Work out the finished part from the listing and answer in its coordinate system (mm). A direction names the side the tool comes from. Coordinates: 2 decimals unless noted, no trailing zeros. Order: outer loops, then holes, each group sorted by start corner. A loop starts at its lowest first (then second) coordinate and runs counter-clockwise, first axis right, second up.
1. Determine the mould class of faces 1 (the cylindrical face through (179.32, 56.47, -0.99)), 2 (the flat face through (92.93, 268, -9)), 3 (the flat face through (-142.93, 268, -9)), 4 (the flat face through (118, 292.93, -9)) for opening direction X: +X half, -X half, draft (parallel to the pull), parting line (faces both ways), or undercut.
2. Find the intervals of material crossed by probe 1 along Y at (x, z) = (0, -10.5); probe 2 along Y at (x, z) = (0, -0.7); probe 3 along Y at (x, z) = (-57, -12.5), in increasing order.
3. A tool of negligible diameter and unlimited length cuts with its end or side. For faces 5 (the cylindrical face through (83.06, -159.69, -12.46)), 6 (the flat face through (-1, 191, 0)), 7 (the flat face through (-70.14, -203.07, -8.87)), 8 (the flat face through (-1, 242.93, -9)), 9 (the flat face through (142.93, 268, -9)), from which of +Z, -Z, +X, -X, +Y, -Y can it reach the whole face along a straight path? Write none if from no direction.
4. Flat-ended cylindrical pins translate along their axes: pin 1 Ø9 at (y, z) = (276.5, -10) entering from +X; pin 2 Ø6 at (x, y) = (3, -127.5) entering from +Z; pin 3 Ø5.5 at (x, z) = (34.5, -5) entering from +Y. Find the tip coordinate at first contact, or state that the pin passes through.
5. The part is cut by section B-B, the plane y = 0. Give the vertices of the cut face in (x, z).
6. The part is cut by section C-C, the plane x = 0. Give the vertices of the cut face in (y, z), then the cut area to 3 significant figures.
Autodesk Inventor part; units mm, degrees
ref_plane "YZ Plane" through (0, 0, 0) normal (1, 0, 0) x (0, 1, 0)
ref_plane "XZ Plane" through (0, 0, 0) normal (0, 1, 0) x (-1, 0, 0)
ref_plane "XY Plane" through (0, 0, 0) normal (0, 0, 1) x (1, 0, 0)
sketch "Sketch1" plane through (0, 0, 0) normal (0, 0, 1) x (1, 0, 0)
  circle A0 centre (0, 0) radius 165
  circle A1 centre (0, 0) radius 175
  line L0 (-192.9296, 192.9296) -> (192.9296, 192.9296)
  line L1 (192.9296, 192.9296) -> (192.9296, -192.9296)
  line L2 (192.9296, -192.9296) -> (-192.9296, -192.9296)
  line L3 (-192.9296, -192.9296) -> (-192.9296, 192.9296)
  line L4 (-192.9296, -192.9296) -> (-178.8933, -212.9296)
  line L5 (-178.8933, -212.9296) -> (178.8933, -212.9296)
  line L6 (178.8933, -212.9296) -> (192.9296, -192.9296)
  line L7 (-192.9296, 192.9296) -> (-142.9296, 242.9296)
  line L8 (-142.9296, 242.9296) -> (142.9296, 242.9296)
  line L9 (142.9296, 242.9296) -> (192.9296, 192.9296)
  line L10 (-142.9296, 242.9296) -> (-92.9296, 242.9296)
  line L11 (-92.9296, 242.9296) -> (-92.9296, 292.9296)
  line L12 (-92.9296, 292.9296) -> (-142.9296, 292.9296)
  line L13 (-142.9296, 292.9296) -> (-142.9296, 242.9296)
  line L14 (142.9296, 242.9296) -> (92.9296, 242.9296)
  line L15 (92.9296, 242.9296) -> (92.9296, 292.9296)
  line L16 (92.9296, 292.9296) -> (142.9296, 292.9296)
  line L17 (142.9296, 292.9296) -> (142.9296, 242.9296)
  line L18 (-60, -212.9296) -> (60, -212.9296)
  line L19 (60, -212.9296) -> (60, -192.9296)
  line L20 (60, -192.9296) -> (-60, -192.9296)
  line L21 (-60, -192.9296) -> (-60, -212.9296)
  circle A2 centre (0, 0) radius 185
  circle A3 centre (0, 0) radius 180
  circle A4 centre (0, 0) radius 188
  point P0 (0, 192.9296)
  point P1 (-192.9296, 0)
  point P2 (0, 242.9296)
  point P3 (0, -212.9296)
  dimension "d0" = 330
  dimension "d1" = 10
  dimension "d2" = 54.938
  dimension "d3" = 54.938
  dimension "d4" = 20
  dimension "d5" = 45
  dimension "d6" = 45
  dimension "d7" = 50
  dimension "d12" = 120
  dimension "d15" = 10
  dimension "d16" = 5
  dimension "d21" = 3
  dimension "d27" = 50
extrude "Extrusion1" add sketch "Sketch1" against normal blind 18 contours A0 | A1 | L7 L8 L9 L0 | L0 L1 L2 L3 | L2 L21 L5 L4 | L13 L12 L11 L8 | L6 L5 L19 L2 | L8 L15 L16 L17 | L2 L19 L5 L21 | A2 | A3 | A4
extrude "Extrusion2" cut sketch "Sketch1" against normal blind 12 contours A0 | A1
extrude "Extrusion3" cut sketch "Sketch1" against normal blind 18 contours L2 L19 L5 L21
extrude "Extrusion4" cut sketch "Sketch1" against normal blind 15 contours A2
extrude "Extrusion5" cut sketch "Sketch1" against normal blind 10 contours A3
extrude "Extrusion6" cut sketch "Sketch1" against normal blind 2 contours A4
chamfer "Chamfer1" distance 20 angle 45 2 edges at (-60, -212.9296, -9) (60, -212.9296, -9)
equation "\"d3\" = d2"
properties part number "Base"
Geometry says:
1. face 1: undercut
1. face 2: undercut
1. face 3: -X half
1. face 4: draft
2. probe 1: y = -192.93 to -185, -180 to -175, 175 to 180, 185 to 242.93
2. probe 2: y = -192.93 to -188, 188 to 242.93
2. probe 3: y = -192.93 to -176, -170.74 to 170.74, 176 to 242.93
3. face 5: +Z
3. face 6: +Z, +X, -X, +Y, -Y
3. face 7: +Z, -Z, -Y
3. face 8: +Z, -Z, +Y
3. face 9: +Z, -Z, +X, +Y
4. pin 1: stops at x = 142.93
4. pin 2: stops at z = -12
4. pin 3: stops at y = 242.93
5. outline: (-192.93, -18) - (192.93, -18) - (192.93, 0) - (188, 0) - (188, -2) - (185, -2) - (185, -15) - (180, -15) - (180, -10) - (175, -10) - (175, -12) - (-175, -12) - (-175, -10) - (-180, -10) - (-180, -15) - (-185, -15) - (-185, -2) - (-188, -2) - (-188, 0) - (-192.93, 0) - close
6. outline: (-192.93, -18) - (242.93, -18) - (242.93, 0) - (188, 0) - (188, -2) - (185, -2) - (185, -15) - (180, -15) - (180, -10) - (175, -10) - (175, -12) - (-175, -12) - (-175, -10) - (-180, -10) - (-180, -15) - (-185, -15) - (-185, -2) - (-188, -2) - (-188, 0) - (-192.93, 0) - close
6. area: 3,380 mm2
